Design review of the part built by this model. Coordinates are the model's own, in mm. Face numbers are marked on the shaded views. Coordinates: 2 decimals unless noted, no trailing zeros. Order: outer loops, then holes, each group sorted by start corner. A loop starts at its lowest first (then second) coordinate and runs counter-clockwise, first axis right, second up. Notation, with made-up numbers: M 23,58 L 61,58 A32 ccw 61,84 Z; hole C 20.25,72 d4. An arc over 180 degrees is marked long. Answer as a JSON object with one key per item and string values.
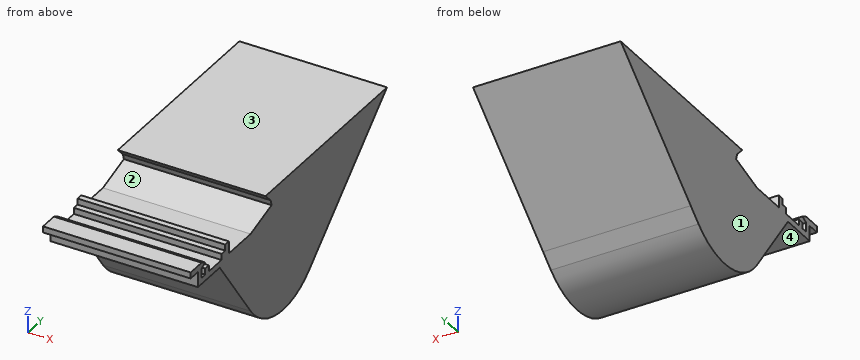
from build123d import *

# Parameters (mm, degrees)
F0_W     = 2
F0_H     = 2
F0_W_2   = 4
F1_DEPTH = 48


with BuildPart() as f1:
    # F0 (on Right) → F1 (new body)
    with BuildSketch(Plane.YZ):
        with BuildLine():
            Line((10.198316, -11.005537), (14.505481, -7.261376))
            Line((14.505481, -7.261376), (-10.490369, 21.493059))
            Line((-10.490369, 21.493059), (-22.027238, 18.191447))
            Line((-22.027238, 18.191447), (-34.027238, 18.191447))
            Line((-34.027238, 18.191447), (-36.027238, 18.191447))
            Line((-36.027238, 18.191447), (-38.027238, 18.191447))
            Line((-38.027238, 18.191447), (-45.027238, 18.191447))
            Line((-45.027238, 18.191447), (-47.027238, 18.191447))
            Line((-47.027238, 18.191447), (-49.027238, 18.191447))
            Line((-49.027238, 18.191447), (-49.027238, 16.191447))
            Line((-49.027238, 16.191447), (-39.027238, 16.191447))
            Line((-39.027238, 16.191447), (-21.926756, -7.345347))
            ThreePointArc((-21.926756, -7.345347), (-6.669481, -16.243127), (10.198316, -11.005537))
        make_face()
        Polygon((53.078913, 26.269997), (-13.84313, 26.269997), (-11.040637, 23.415871), (-10.490369, 21.493059), (14.505481, -7.261376), align=None)
        Polygon((-36.027238, 18.191447), (-34.027238, 18.191447), (-34.027238, 22.191447), (-36.027238, 22.191447), (-36.027238, 20.191447), align=None)
        with Locations((-37.027238, 19.191447)):
            Rectangle(F0_W, F0_H)
        with Locations((-46.027238, 19.191447)):
            Rectangle(F0_W, F0_H)
        Polygon((-51.027238, 16.191447), (-49.027238, 16.191447), (-49.027238, 18.191447), (-49.027238, 21.191447), (-49.027238, 22.191447), (-49.027238, 23.191447), (-51.027238, 23.191447), (-51.027238, 21.191447), align=None)
        Polygon((-49.027238, 22.191447), (-49.027238, 21.191447), (-47.027238, 22.191447), align=None)
        Polygon((-49.027238, 23.191447), (-49.027238, 22.191447), (-47.027238, 22.191447), align=None)
        with Locations((-53.027238, 22.191447)):
            Rectangle(F0_W_2, F0_H)
    extrude(amount=F1_DEPTH)


solid = f1.part
1) Add section A-A (x = 9.5). State the section outline as (y, z) points, and give its area (3 significant figures).
Taken from the geometry:
{"outline": "M -55.03,21.19 L -51.03,21.19 L -51.03,16.19 L -39.03,16.19 L -21.93,-7.35 A21.93 ccw 10.2,-11.01 L 53.08,26.27 L -13.84,26.27 L -11.04,23.42 L -10.49,21.49 L -22.03,18.19 L -34.03,18.19 L -34.03,22.19 L -36.03,22.19 L -36.03,20.19 L -38.03,20.19 L -38.03,18.19 L -45.03,18.19 L -45.03,20.19 L -47.03,20.19 L -47.03,18.19 L -49.03,18.19 L -49.03,21.19 L -47.03,22.19 L -49.03,23.19 L -55.03,23.19 Z", "area": "2,330 mm2"}
2) Add section C-C (z = 5.5). State the section outline as (x, y) points, and give its area (3 significant figures).
Taken from the geometry:
{"outline": "M 0,-31.26 L 48,-31.26 L 48,29.19 L 0,29.19 Z", "area": "2,900 mm2"}
3) Add section B-B (y = 23.5). State the section outline as (x, z) points, and give its area (3 significant figures).
Taken from the geometry:
{"outline": "M 0,0.56 L 48,0.56 L 48,26.27 L 0,26.27 Z", "area": "1,230 mm2"}
4) Mouldability with a two-part tool opening along Z and no side actions: class the marked faces 1, 2, 3 and 4 as released by +Z, released by -Z, zero draft, split by the parting line, or undercut.
Taken from the geometry:
{"face 1": "zero draft", "face 2": "undercut", "face 3": "released by +Z", "face 4": "released by -Z"}
5) To check wall thickness, follow L1, parallel to Y at x = 45, z = 22; L2, parallel to Z at x = 33, y = -42; L3, parallel to Z at x = 38, y = -8.5. State the ranges of each line that lie inside material, in increasing order.
Taken from the geometry:
{"L1": "y = -55.03 to -47.41, -36.03 to -34.03, -10.64 to 48.17", "L2": "z = 16.19 to 18.19", "L3": "z = -15.96 to 26.27"}
6) Insertion check: pin 1 Ø8 at (x, z) = (39.5, 3) entering from +Y; pin 2 Ø3.5 at (x, z) = (20, 20) entering from +Y; pin 3 Ø3 at (x, y) = (31, -22) entering from -Z. Each pin has a flat end and moves straight along its axis. Give the tip position at first contact, or say it passes through.
Taken from the geometry:
{"pin 1": "stops at y = 30.91", "pin 2": "stops at y = 47.88", "pin 3": "stops at z = -9.11"}
